```python
from build123d import *

# Parameters (mm, degrees)
SKETCH_1_W                      = 4
SKETCH_1_H                      = 49.98
RIGHT_RF_PLATE_DEPTH            = 8.851909566
SKETCH_2_R                      = 0.8
FRAME_2XD1P6_THROUGH_DEPTH      = 72.016485431
SKETCH_3_R                      = 2.05
SMA_CENTER_D4P1_DEPTH           = 4
SKETCH_4_R                      = 0.875
SMA_UPPER_2XD1P75_THROUGH_DEPTH = 48.179152176
SKETCH_5_W                      = 6.7
SKETCH_5_H                      = 11.5
TYPEC_WINDOW_11P5X6P7_DEPTH     = 4


with BuildPart() as part:
    # 草图1 → Right_RF_Plate (new body)
    with BuildSketch(Plane.XY):
        with Locations((51.65, 20.69)):
            Rectangle(SKETCH_1_W, SKETCH_1_H)
    extrude(amount=RIGHT_RF_PLATE_DEPTH)


with BuildPart() as part_1:
    # Stock_Z_Position: moved
    add(part.part.moved(Location((0, 0, 2.248090434))))

    # 草图2 → Frame_2xD1p6_Through (cut, through all)
    with BuildSketch(Plane.XY.offset(11.1)):
        with Locations((51.65, -1)):
            Circle(SKETCH_2_R)
        with Locations((51.65, 43)):
            Circle(SKETCH_2_R)
    extrude(amount=-FRAME_2XD1P6_THROUGH_DEPTH, mode=Mode.SUBTRACT)

    # 草图3 → SMA_Center_D4p1 (cut)
    with BuildSketch(Plane(origin=(53.65, 0, 0), x_dir=(0, 0, -1), z_dir=(1, 0, 0))):
        with Locations((-3.899496327, 10.725)):
            Circle(SKETCH_3_R)
    extrude(amount=-SMA_CENTER_D4P1_DEPTH, mode=Mode.SUBTRACT)

    # 草图4 → SMA_Upper_2xD1p75_Through (cut, through all)
    with BuildSketch(Plane(origin=(53.65, 0, 0), x_dir=(0, 0, -1), z_dir=(1, 0, 0))):
        with Locations((-8.199496327, 6.425)):
            Circle(SKETCH_4_R)
        with Locations((-8.199496327, 15.025)):
            Circle(SKETCH_4_R)
    extrude(amount=-SMA_UPPER_2XD1P75_THROUGH_DEPTH, mode=Mode.SUBTRACT)

    # 草图5 → TypeC_Window_11p5x6p7 (cut)
    with BuildSketch(Plane(origin=(53.65, 0, 0), x_dir=(0, 0, -1), z_dir=(1, 0, 0))):
        with Locations((-4.25, 31.65)):
            Rectangle(SKETCH_5_W, SKETCH_5_H)
    extrude(amount=-TYPEC_WINDOW_11P5X6P7_DEPTH, mode=Mode.SUBTRACT)


solid = part_1.part
```
For this review, take the finished solid that the model builds, in its own axes (mm). A direction names the side the tool comes from. Coordinates: 2 decimals unless noted, no trailing zeros. Write each loop counter-clockwise with the first axis right and the second up, starting at its lowest first coordinate (ties: lowest second). Pieces come first, ordered by that corner, then holes. Notation, with made-up numbers: (-15.75, 76.25) - (-1.75, 76.25) arc R24 ccw to (-1.75, 96.25) - close; hole circle Ø6 at (-21.75, 8). An arc over 180 degrees is marked (long way). Answer in a Markdown table with one row per item. Add a question column.
Q1. We need section C-C, the plane z = 10.25. State the section outline as (x, y) points, and give its area (3 significant figures).
Q2. Draft analysis for pull direction Y (two halves, no side actions). For faces 3 (the cylindrical face through (51.68, 15.62, 8.84)), 4 (the flat face through (52, -4.3, 7)), 5 (the flat face through (53.65, 20, 7)), state which applies: +Y half, -Y half, draft (parallel to the pull), parting line (faces both ways), or undercut.
Q3. We need section B-B, the plane x = 51.55. Count the separate pieces of the cut face and the enclosed holes in it, and give its area (3 significant figures).
Q4. We need section D-D, the plane y = 6. State the section outline as (x, z) points.
Q5. Tool access review of faces 1 (the flat face through (52, 45.68, 7)), 2 (the flat face through (52, 25.9, 5)): name each direction out of +Z, -Z, +X, -X, +Y, -Y from which nothing blocks a thin tool from reaching the whole face with its end or side.
Q6. We need section A-A, the plane y = 43. State the section outline as (x, z) points.
Q7. For P1, Ø2, axis at x = 51.5, y = 31, coming from the -Z side, flat-tipped, find the tip position at first contact; note if it passes through.
Q8. For probe 1 along Y at (x, z) = (52, 7.75); probe 2 along Y at (x, z) = (51.8, 8.75); probe 3 along Y at (x, z) = (50.6, 5), list the stretches that pass through material, from the lowest coordinate up.
Answer list:
| question | item | result |
|---|---|---|
| 1 | outline | (49.65, -4.3) - (53.65, -4.3) - (53.65, 45.68) - (49.65, 45.68) - close; hole circle Ø1.6 at (51.65, -1); hole circle Ø1.6 at (51.65, 43) |
| 1 | area | 196 mm2 |
| 2 | face 3 | undercut |
| 2 | face 4 | -Y half |
| 2 | face 5 | draft |
| 3 | separate pieces | 3 |
| 3 | enclosed holes | 2 |
| 3 | area | 335 mm2 |
| 4 | outline | (49.65, 2.25) - (53.65, 2.25) - (53.65, 7.43) - (49.65, 7.43) - close; (49.65, 8.96) - (53.65, 8.96) - (53.65, 11.1) - (49.65, 11.1) - close |
| 5 | face 1 | +Z, -Z, +X, -X, +Y |
| 5 | face 2 | -Z, +X, -X |
| 6 | outline | (49.65, 2.25) - (50.85, 2.25) - (50.85, 11.1) - (49.65, 11.1) - close; (52.45, 2.25) - (53.65, 2.25) - (53.65, 11.1) - (52.45, 11.1) - close |
| 7 | P1 | stops at z = 7.6 |
| 8 | probe 1 | y = -4.3 to -1.72, -0.28 to 5.67, 7.18 to 14.27, 15.78 to 42.28, 43.72 to 45.68 |
| 8 | probe 2 | y = -4.3 to -1.79, -0.21 to 5.74, 7.11 to 14.34, 15.71 to 42.21, 43.79 to 45.68 |
| 8 | probe 3 | y = -4.3 to 9, 12.45 to 25.9, 37.4 to 45.68 |
